Input: part model. Units: mm. Frame: model coordinates. A direction names the side the tool comes from. Round coordinates to 2 decimals unless told otherwise and drop trailing zeros. Loops run counter-clockwise (first coordinate to the right, second up) from the corner with the lowest first, then second, coordinate; pieces in that order, holes last. Notation, with made-up numbers: M 14,-36.75 L 55,-36.75 A18 ccw 55,-10.75 Z; hole C -19.75,16.5 d1. An arc over 180 degrees is marked long. Return JSON: item names as keys, results as strings. Group by question number.
1) Mould query, pull axis X, two halves, no side actions, for faces 1 (the face through (-0.052, 14.165, -4.69)), 2 (the face through (-0.07, 11.92, -4.43)), 3 (the face through (3.816, 16.864, 4.045)), 4 (the face through (0, 17, -3.533)). Classes: +X half, -X half, draft (parallel to the pull), parting line (faces both ways), or undercut.
2) Contact query for flat-ended pins moving along their axis: P1, Ø5.5, axis at y = 29.5, z = 0.5, coming from the +X side; P2, Ø3, axis at x = 2.5, z = 0.5, coming from the -Y side; P3, Ø5, axis at x = 3.5, z = 4.5, coming from the -Y side. Output: stop coordinate, or through.
3) Section C-C (y = 16.25). Output: boundary loops of the cut face in (x, z), plus the area to 3 significant figures.
4) Section D-D (z = 4.5). Output: boundary loops of the cut face in (x, y).
5) Section A-A (y = 19). Output: boundary loops of the cut face in (x, z), plus the area to 3 significant figures.
6) Access query for faces 5 (the face through (3.337, 28, 0)), 6 (the face through (0, 17, 3.533)), 7 (the face through (-2.252, 19.178, 5.432)), 8 (the face through (-3.337, 28, 0)). Directions: +Z, -Z, +X, -X, +Y, -Y. A direction counts if a zero-diameter tool reaches every point of the face in a straight line with its end or side. Return the directions, or none.
7) Section B-B (x = 0). Output: boundary loops of the cut face in (y, z).
8) Material intervals for line 1 (Y direction, x = 0, z = -4.7); line 2 (Z direction, x = -4, y = 19.5); line 3 (Z direction, x = -3.5, y = 19.25), sorted ascending. Write a range as from..to.
from build123d import *

# Parameters (mm, degrees)
SKETCH1_R           = 12
BOSS_EXTRUDE1_DEPTH = 33.53
CUT_EXTRUDE1_DEPTH  = 19.6
CHAMFER1_SIZE       = 0.4
SKETCH3_R           = 9.375
CUT_EXTRUDE2_DEPTH  = 3.4
CUT_EXTRUDE2_DRAFT  = -35
SKETCH4_W           = 24
SKETCH4_H           = 14.42225279
CUT_EXTRUDE3_DEPTH  = 17.4
SKETCH5_R           = 2.415
CUT_EXTRUDE4_DEPTH  = 33.7
CUT_EXTRUDE5_START  = -9
SKETCH6_R           = 12
CUT_EXTRUDE5_DEPTH  = 9
BOSS_EXTRUDE2_START = -7.13
SKETCH7_R           = 12
BOSS_EXTRUDE2_DEPTH = 7.13
SKETCH8_W           = 13.62
SKETCH8_H           = 13.62
BOSS_EXTRUDE3_DEPTH = 17.8
CHAMFER2_SIZE       = 0.5
SCALE1_SCALE        = 0.49


with BuildPart() as part:
    # Sketch1 → Boss-Extrude1 (new body)
    with BuildSketch(Plane(origin=(0, 0, 0), x_dir=(1, 0, 0), z_dir=(0, 1, 0))):
        with Locations(Location((0, 0, 0), (0, 0, 270))):
            Circle(SKETCH1_R)
    extrude(amount=BOSS_EXTRUDE1_DEPTH)

    # Sketch2 → Cut-Extrude1 (cut)
    with BuildSketch(Plane(origin=(0, 33.53, 0), x_dir=(1, 0, 0), z_dir=(0, 1, 0))):
        with BuildLine():
            Line((-6.5, 6.5), (-2.5, 6.5))
            ThreePointArc((-2.5, 6.5), (0, 7.211126395), (2.5, 6.5))
            Line((2.5, 6.5), (6.5, 6.5))
            Line((6.5, 6.5), (6.5, 2.5))
            ThreePointArc((6.5, 2.5), (7.211126395, 0), (6.5, -2.5))
            Line((6.5, -2.5), (6.5, -6.5))
            Line((6.5, -6.5), (2.5, -6.5))
            ThreePointArc((2.5, -6.5), (0, -7.211126395), (-2.5, -6.5))
            Line((-2.5, -6.5), (-6.5, -6.5))
            Line((-6.5, -6.5), (-6.5, -2.5))
            ThreePointArc((-6.5, -2.5), (-7.211126395, 0), (-6.5, 2.5))
            Line((-6.5, 2.5), (-6.5, 6.5))
        make_face()
    extrude(amount=-CUT_EXTRUDE1_DEPTH, mode=Mode.SUBTRACT)

    # Chamfer1
    chamfer1_edges = [part.edges().sort_by_distance(p)[0] for p in [
        (-6.5, 23.73, -6.5),
        (6.5, 23.73, -6.5),
        (6.5, 23.73, 6.5),
        (-6.5, 23.73, 6.5),
    ]]
    chamfer(chamfer1_edges, length=CHAMFER1_SIZE)


with BuildPart() as cut_extrude2_tool:
    # Sketch3 → Cut-Extrude2 (with draft: the straight prism first)
    with BuildSketch(Plane(origin=(0, 33.53, 0), x_dir=(1, 0, 0), z_dir=(0, 1, 0))):
        Circle(SKETCH3_R)
    extrude(amount=-CUT_EXTRUDE2_DEPTH)
    # Cut-Extrude2: the draft: its side faces are tilted about the plane it starts from
    cut_extrude2_sides = [cut_extrude2_tool.faces().sort_by_distance(p)[0] for p in [
        (-9.375, 31.83, 0),
    ]]
    draft(cut_extrude2_sides, Plane(origin=(0, 33.53, 0), x_dir=(1, 0, 0), z_dir=(0, 1, 0)), CUT_EXTRUDE2_DRAFT)


with BuildPart() as part_1:
    add(part.part)

    # Cut-Extrude2: cut by cut_extrude2_tool
    add(cut_extrude2_tool.part, mode=Mode.SUBTRACT)

    # Sketch4 → Cut-Extrude3 (cut)
    with BuildSketch(Plane.XZ):
        Rectangle(SKETCH4_W, SKETCH4_H)
    extrude(amount=-CUT_EXTRUDE3_DEPTH, mode=Mode.SUBTRACT)

    # Sketch5 → Cut-Extrude4 (cut, symmetric)
    with BuildSketch(Plane.XY):
        with Locations(Location((0, 7, 0), (0, 0, 90))):
            Circle(SKETCH5_R)
        with BuildLine():
            ThreePointArc((-6.854820161, 5.581747356), (0, 0), (6.854820161, 5.581747356))
            Line((6.854820161, 5.581747356), (9.3, 17.4))
            Line((9.3, 17.4), (12, 17.4))
            Line((12, 17.4), (12, -3.192277431))
            Line((12, -3.192277431), (-12, -3.192277431))
            Line((-12, -3.192277431), (-12, 17.4))
            Line((-12, 17.4), (-9.3, 17.4))
            Line((-9.3, 17.4), (-6.854820161, 5.581747356))
        make_face()
    extrude(amount=CUT_EXTRUDE4_DEPTH, both=True, mode=Mode.SUBTRACT)

    # Sketch6 → Cut-Extrude5 (cut)
    with BuildSketch(Plane(origin=(0, 33.53, 0), x_dir=(1, 0, 0), z_dir=(0, 1, 0)).offset(CUT_EXTRUDE5_START)):
        with Locations(Location((0, 0, 0), (0, 0, 55.16360803))):
            Circle(SKETCH6_R)
    extrude(amount=CUT_EXTRUDE5_DEPTH, mode=Mode.SUBTRACT)

    # Sketch7 → Boss-Extrude2 (add)
    with BuildSketch(Plane(origin=(0, 24.53, 0), x_dir=(1, 0, 0), z_dir=(0, 1, 0)).offset(BOSS_EXTRUDE2_START)):
        with Locations(Location((0, 0, 0), (0, 0, 55.16360803))):
            Circle(SKETCH7_R)
    extrude(amount=BOSS_EXTRUDE2_DEPTH)

    # Sketch8 → Boss-Extrude3 (add)
    with BuildSketch(Plane(origin=(0, 24.53, 0), x_dir=(1, 0, 0), z_dir=(0, 1, 0))):
        Rectangle(SKETCH8_W, SKETCH8_H)
    extrude(amount=BOSS_EXTRUDE3_DEPTH)

    # Sketch9 → Cut-Revolve1 (revolve, cut)
    with BuildSketch(Plane.XY, mode=Mode.PRIVATE) as cut_revolve1_sk:
        Polygon((5.7, 42.33), (13.111265215, 42.33), (13.111265215, 34.918734785), align=None)
    revolve(cut_revolve1_sk.sketch.rotate(Axis((0, 44.4465, 0), (0, -1, 0)), 304.83639197), axis=Axis((0, 44.4465, 0), (0, -1, 0)), mode=Mode.SUBTRACT)

    # Chamfer2
    chamfer2_edges = [part_1.edges().sort_by_distance(p)[0] for p in [
        (6.81, 24.53, 0),
        (0, 24.53, -6.81),
        (-6.81, 24.53, 0),
        (0, 24.53, 6.81),
    ]]
    chamfer(chamfer2_edges, length=CHAMFER2_SIZE)

    # Sketch10 → Revolve1 (revolve)
    with BuildSketch(Plane(origin=(0, 0, 0), x_dir=(0, 0, -1), z_dir=(1, 0, 0))):
        with BuildLine():
            Line((6.81, 34.73), (6.81, 31.73))
            ThreePointArc((6.81, 31.73), (7.806952033, 33.085121585), (8.16, 34.73))
            Line((8.16, 34.73), (6.81, 34.73))
        make_face()
    revolve1 = revolve(axis=Axis((0, 34.73, -6.81), (0, 0, -1)))

    # Mirror1: Revolve1 across plane
    add(revolve1.mirror(Plane.XY))


with BuildPart() as part_2:
    # Scale1: scaled about (-1.67e-07, 23.367427714, 2.93e-06)
    add(part_1.part.scale(SCALE1_SCALE).moved(Location((-8.5e-08, 11.917388134, 1.494e-06))))


solid = part_2.part
Returned:
{
 "1": {"face 1": "undercut", "face 2": "parting line", "face 3": "+X half", "face 4": "draft"},
 "2": {"P1": "stops at x = 3.34", "P2": "stops at y = 20.44", "P3": "stops at y = 12.07"},
 "3": {"outline": "M -3.69,-4.58 A5.88 ccw -0.77,-5.83 L -0.77,-3.53 L -3.69,-3.53 Z; M -3.69,3.53 L -0.77,3.53 L -0.77,5.83 A5.88 ccw -3.69,4.58 Z; M 0.77,-5.83 A5.88 ccw 3.69,-4.58 L 3.69,-3.53 L 0.77,-3.53 Z; M 0.77,3.53 L 3.69,3.53 L 3.69,4.58 A5.88 ccw 0.77,5.83 Z", "area": "21.4 mm^2"},
 "4": {"outline": "M -3.78,16.71 L -3.36,14.65 A3.43 ccw 3.36,14.65 L 3.78,16.71 L 3.78,23.94 L -3.78,23.94 Z; hole C 0,15.35 d2.37"},
 "5": {"outline": "M -4.26,-4.05 A5.88 ccw 4.26,-4.05 L 4.26,-3.53 L -4.26,-3.53 Z; M -4.26,3.53 L 4.26,3.53 L 4.26,4.05 A5.88 ccw -4.26,4.05 Z", "area": "30.3 mm^2"},
 "6": {"face 5": "+Z, -Z, +X, +Y", "face 6": "+X, -X, -Y", "face 7": "+Y, -Y", "face 8": "+Z, -Z, -X, +Y"},
 "7": {"outline": "M 11.92,-5.88 L 14.16,-5.88 L 14.16,-3.53 L 11.92,-3.53 Z; M 11.92,3.53 L 14.16,3.53 L 14.16,5.88 L 11.92,5.88 Z; M 16.53,-5.88 L 23.94,-5.88 L 23.94,-3.58 L 24.18,-3.34 L 27.47,-3.34 A1.96 ccw 30.41,-3.34 L 32.12,-3.34 L 32.66,-2.79 L 32.66,2.79 L 32.12,3.34 L 30.41,3.34 A1.96 ccw 27.47,3.34 L 24.18,3.34 L 23.94,3.58 L 23.94,5.88 L 16.53,5.88 L 16.53,3.53 L 20.44,3.53 L 20.44,-3.53 L 16.53,-3.53 Z"},
 "8": {"line 1": "y = 11.92..14.16, 16.53..23.94", "line 2": "z = -4.31..-3.53, 3.53..4.31", "line 3": "z = -4.72..-3.53, 3.53..4.72"}
}
